from build123d import *

# Parameters (mm, degrees)
SKETCH_1_R          = 42
SKETCH_1_R_2        = 1.5
SKETCH_1_R_3        = 22.5
EXTRUDE_1_DEPTH     = 5
SKETCH_1_4_R        = 32.6
CUT_EXTRUDE_1_DEPTH = 2


with BuildPart() as part:
    # Sketch 1 → Extrude 1 (new body)
    with BuildSketch(Plane.XY):
        Circle(SKETCH_1_R)
        with Locations((0, 37.5)):
            Circle(SKETCH_1_R_2, mode=Mode.SUBTRACT)
        with Locations((-37.5, 0)):
            Circle(SKETCH_1_R_2, mode=Mode.SUBTRACT)
        with Locations((37.5, 0)):
            Circle(SKETCH_1_R_2, mode=Mode.SUBTRACT)
        Circle(SKETCH_1_R_3, mode=Mode.SUBTRACT)
        with Locations((0, -37.5)):
            Circle(SKETCH_1_R_2, mode=Mode.SUBTRACT)
    extrude(amount=EXTRUDE_1_DEPTH)

    # Sketch 1_4 → Cut-Extrude 1 (cut)
    with BuildSketch(Plane.XY):
        Circle(SKETCH_1_4_R)
    extrude(amount=CUT_EXTRUDE_1_DEPTH, mode=Mode.SUBTRACT)


solid = part.part
Build history of the part. All positions in model axes, mm. A direction names the side the tool comes from. Round coordinates to 2 decimals unless told otherwise and drop trailing zeros. Write each loop counter-clockwise with the first axis right and the second up, starting at its lowest first coordinate (ties: lowest second). Pieces come first, ordered by that corner, then holes. Notation, with made-up numbers: M 23,89.25 L 65,89.25 A24 cw 65,108.25 Z; hole C 89.25,32.5 d7. An arc over 180 degrees is marked long. Answer in a Markdown table with one row per item.
1. Mould opens along Y. For faces 3 (the face through (-25.9, -19.8, 1)), 4 (the face through (22, -25, 0)), 5 (the face through (40.06, 12.62, 2.46)) say: +Y half, -Y half, draft (parallel to the pull), parting line (faces both ways), or undercut.
Geometry check:
| item | result |
|---|---|
| face 3 | undercut |
| face 4 | draft |
| face 5 | parting line |
2. Saw through at B-B (x = 0). List the corners of the cut face in (y, z).
Geometry check:
| item | result |
|---|---|
| outline | M -42,0 L -39,0 L -39,5 L -42,5 Z; M -36,0 L -32.6,0 L -32.6,2 L -22.5,2 L -22.5,5 L -36,5 Z; M 22.5,2 L 32.6,2 L 32.6,0 L 36,0 L 36,5 L 22.5,5 Z; M 39,0 L 42,0 L 42,5 L 39,5 Z |
3. Saw through at A-A (x = 37.5). List the corners of the cut face in (y, z), and give its area (3 significant figures).
Geometry check:
| item | result |
|---|---|
| outline | M -18.91,0 L -1.5,0 L -1.5,5 L -18.91,5 Z; M 1.5,0 L 18.91,0 L 18.91,5 L 1.5,5 Z |
| area | 174 mm2 |
4. Probe L1, parallel to Y at x = 0, z = 0.7; L2, parallel to Y at x = 0, z = 3.15; L3, parallel to Y at x = 15, z = 1. List the from-to ranges inside material, lowest first. Write a range as [from, to].
Geometry check:
| item | result |
|---|---|
| L1 | [-42, -39], [-36, -32.6], [32.6, 36], [39, 42] |
| L2 | [-42, -39], [-36, -22.5], [22.5, 36], [39, 42] |
| L3 | [-39.23, -28.94], [28.94, 39.23] |
5. Which spindle directions (+Z, -Z, +X, -X, +Y, -Y) get a long thin tool onto all of the face, cutting with end or side? Do faces 1 (the face through (36.3, -0.9, 2.5)), 2 (the face through (7, 22, 2)). Say none if no direction does.
Geometry check:
| item | result |
|---|---|
| face 1 | +Z, -Z |
| face 2 | -Z |
6. Saw through at C-C (z = 1.05). List the corners of the cut face in (x, y), and give its area (3 significant figures).
Geometry check:
| item | result |
|---|---|
| outline | C 0,0 d84; hole C -37.5,0 d3; hole C 0,0 d65.2; hole C 0,-37.5 d3; hole C 0,37.5 d3; hole C 37.5,0 d3 |
| area | 2,170 mm2 |
7. Flat gauge pins, fed straight in: P1, Ø2, axis at y = -9.5, z = 2.5, coming from the -X side; P2, Ø2, axis at x = -11.5, z = 4.5, coming from the +Y side; P3, Ø2.5, axis at x = 37.5, y = 0, coming from the +Z side; P4, Ø3, axis at y = -15.5, z = 3.5, coming from the -X side. Where does each tip first touch, or does it go through?
Geometry check:
| item | result |
|---|---|
| P1 | x = -41.13 |
| P2 | y = 40.67 |
| P3 | through |
| P4 | x = -39.6 |
